The listing builds one solid part. Answer for the finished solid, in the listing's coordinates (mm). A direction names the side the tool comes from. Give positions to 0.01 mm unless a question says otherwise; leave off trailing zeros. Loops run counter-clockwise (first coordinate to the right, second up) from the corner with the lowest first, then second, coordinate; pieces in that order, holes last. Notation, with made-up numbers: M 38.25,72.5 L 61.25,72.5 A6 ccw 61.25,81.5 Z; hole C 88.25,80.25 d4. An arc over 180 degrees is marked long. Return JSON: item names as keys, results as strings.
from build123d import *

# Parameters (mm, degrees)
SKETCH1_R           = 15
BOSS_EXTRUDE1_DEPTH = 58
SKETCH4_W           = 35
SKETCH4_H           = 6
BOSS_EXTRUDE3_DEPTH = 3
SKETCH5_W           = 3
SKETCH5_H           = 6
BOSS_EXTRUDE4_DEPTH = 5
SKETCH6_R           = 2.5
BOSS_EXTRUDE5_DEPTH = 17.5


with BuildPart() as part:
    # Sketch1 → Boss-Extrude1 (new body)
    with BuildSketch(Plane(origin=(0, 0, 0), x_dir=(1, 0, 0), z_dir=(0, 1, 0))):
        with Locations(Location((0, 0, 0), (0, 0, 90))):
            Circle(SKETCH1_R)
    extrude(amount=BOSS_EXTRUDE1_DEPTH)

    # Sketch4 → Boss-Extrude3 (add)
    with BuildSketch(Plane(origin=(0, 58, 0), x_dir=(1, 0, 0), z_dir=(0, 1, 0))):
        Rectangle(SKETCH4_W, SKETCH4_H)
    extrude(amount=BOSS_EXTRUDE3_DEPTH)

    # Sketch5 → Boss-Extrude4 (add)
    with BuildSketch(Plane(origin=(0, 61, 0), x_dir=(1, 0, 0), z_dir=(0, 1, 0))):
        with Locations((-15.95745503, 0)):
            Rectangle(SKETCH5_W, SKETCH5_H)
    boss_extrude4 = extrude(amount=BOSS_EXTRUDE4_DEPTH)

    # Mirror2: Boss-Extrude4 across plane
    add(boss_extrude4.mirror(Plane(origin=(0, 0, 0), x_dir=(0, 0, 1), z_dir=(1, 0, 0))))

    # Sketch6 → Boss-Extrude5 (add)
    with BuildSketch(Plane(origin=(0, 0, 0), x_dir=(0, 0, -1), z_dir=(1, 0, 0))):
        with Locations(Location((0, 2.5, 0), (0, 0, 270))):
            Circle(SKETCH6_R)
    boss_extrude5 = extrude(amount=BOSS_EXTRUDE5_DEPTH)

    # Mirror3: Boss-Extrude5 across plane
    add(boss_extrude5.mirror(Plane(origin=(0, 0, 0), x_dir=(0, 0, 1), z_dir=(1, 0, 0))))


solid = part.part
(1) Straight lines are drawn through the part: line 1 along Y through (x, z) = (-0.5, 9); line 2 along Y through (x, z) = (4, -1); line 3 along Z through (x, y) = (4, 51). For each, find the intervals that lie inside material, in ascending order.
Values follow:
{"line 1": "0 to 58", "line 2": "0 to 61", "line 3": "-14.46 to 14.46"}
(2) Determine the mould class of faces 5 (the flat face through (0, 0, 0)), 6 (the flat face through (-14.457, 63, 0)), 7 (the cylindrical face through (16.13, 2.83, -2.48)) for opening direction Y: released by +Y, released by -Y, zero draft, split by the parting line, or undercut.
Values follow:
{"face 5": "released by -Y", "face 6": "zero draft", "face 7": "undercut"}
(3) Given pin 1 (5.5 mm diameter, centred on y = 64.5, z = -1, fed in from -X); pin 2 (2 mm diameter, centred on x = -6.5, y = 34.5, fed in from +Z); pin 3 (5 mm diameter, centred on x = -4, z = 1, fed in from +Y), each flat-ended and moving along its own axis, determine where each tip first touches the part or whether it passes through.
Values follow:
{"pin 1": "x = -17.46", "pin 2": "z = 13.96", "pin 3": "y = 61"}
(4) The part is cut by section C-C (y = 13.5). Determine the outline of the cut face in (x, z), and give its area (3 significant figures).
Values follow:
{"outline": "C 0,0 d30", "area": "707 mm²"}
(5) The part is cut by section B-B (y = 2.5). Determine the outline of the cut face in (x, z).
Values follow:
{"outline": "M -17.5,-2.5 L -14.79,-2.5 A15 ccw 14.79,-2.5 L 17.5,-2.5 L 17.5,2.5 L 14.79,2.5 A15 ccw -14.79,2.5 L -17.5,2.5 Z"}
(6) A tool of negligible diameter and unlimited length cuts with its end or side. For faces 1 (the flat face through (14.457, 63, 0)), 2 (the flat face through (0, 60, -3)), 3 (the cylindrical face through (-16.13, 2.83, -2.48)), 4 (the flat face through (0, 60, 3)), from which of +Z, -Z, +X, -X, +Y, -Y can it reach the whole face along a straight path? Write none if from no direction.
Values follow:
{"face 1": "+Z, -Z, +Y", "face 2": "-Z, +X, -X, +Y", "face 3": "-X", "face 4": "+Z, +X, -X, +Y"}
(7) The part is cut by section A-A (x = 0). Determine the outline of the cut face in (y, z), and give its area (3 significant figures).
Values follow:
{"outline": "M 0,-15 L 58,-15 L 58,-3 L 61,-3 L 61,3 L 58,3 L 58,15 L 0,15 Z", "area": "1,760 mm²"}
(8) The part is cut by section D-D (z = 5.5). Determine the outline of the cut face in (x, y).
Values follow:
{"outline": "M -13.96,0 L 13.96,0 L 13.96,58 L -13.96,58 Z"}
